from build123d import *

# Parameters (mm, degrees)
SKETCH1_W           = 165
SKETCH1_H           = 50
BOSS_EXTRUDE1_DEPTH = 2.5
FILLET1_R           = 25
SKETCH2_R           = 2.5
CUT_EXTRUDE1_DEPTH  = 2.5
SKETCH3_R           = 2.5
CUT_EXTRUDE2_DEPTH  = 2.5
SKETCH4_R           = 2.25
BOSS_EXTRUDE2_DEPTH = 8
SKETCH6_R           = 1.5
CUT_EXTRUDE4_DEPTH  = 87.841810207


with BuildPart() as part:
    # Sketch1 → Boss-Extrude1 (new body)
    with BuildSketch(Plane.XY):
        Rectangle(SKETCH1_W, SKETCH1_H)
    extrude(amount=BOSS_EXTRUDE1_DEPTH)

    # Fillet1
    fillet1_edges = [part.edges().sort_by_distance(p)[0] for p in [
        (-82.5, -25, 1.25),
        (-82.5, 25, 1.25),
        (82.5, -25, 1.25),
        (82.5, 25, 1.25),
    ]]
    fillet(fillet1_edges, radius=FILLET1_R - 0.0001)  # a hair under: the kernel refuses the full size

    # Sketch2 → Cut-Extrude1 (cut)
    with BuildSketch(Plane.XY.offset(2.5)):
        with Locations((-5, 16)):
            Circle(SKETCH2_R)
        with Locations((5, 16)):
            Circle(SKETCH2_R)
    cut_extrude1 = extrude(amount=-CUT_EXTRUDE1_DEPTH, mode=Mode.SUBTRACT)

    # Mirror1: Cut-Extrude1 across plane
    add(cut_extrude1.mirror(Plane.ZX), mode=Mode.SUBTRACT)

    # Sketch3 → Cut-Extrude2 (cut)
    with BuildSketch(Plane(origin=(0, 0, 0), x_dir=(-1, 0, 0), z_dir=(0, 0, -1))):
        with Locations((-57.5, 0)):
            Circle(SKETCH3_R)
    extrude(amount=-CUT_EXTRUDE2_DEPTH, mode=Mode.SUBTRACT)

    # Sketch4 → Boss-Extrude2 (add)
    with BuildSketch(Plane.XY.offset(2.5)):
        with Locations(Location((-57.5, 0, 0), (0, 0, 180))):
            Circle(SKETCH4_R)
    extrude(amount=BOSS_EXTRUDE2_DEPTH)

    # Sketch6 → Cut-Extrude4 (cut, through all)
    with BuildSketch(Plane(origin=(0, 0, 0), x_dir=(-1, 0, 0), z_dir=(0, 0, -1))):
        with Locations((-25, 18.5)):
            Circle(SKETCH6_R)
        with Locations((25, 18.5)):
            Circle(SKETCH6_R)
    extrude(amount=-CUT_EXTRUDE4_DEPTH, mode=Mode.SUBTRACT)


solid = part.part
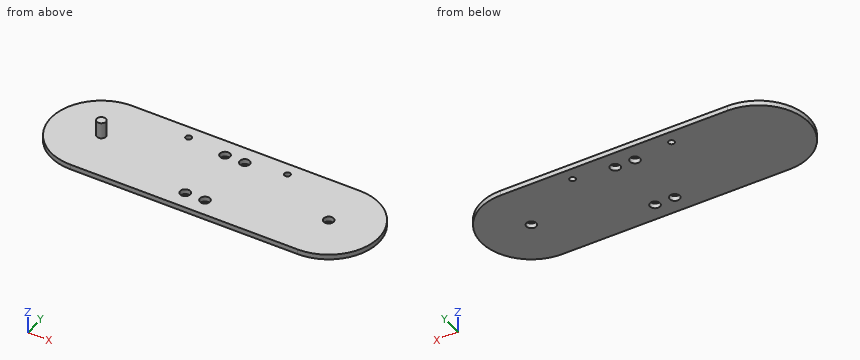
Could you check a few things on this model? Use its own coordinates, in mm. Round coordinates to 2 decimals unless told otherwise and drop trailing zeros. Write each loop counter-clockwise with the first axis right and the second up, starting at its lowest first coordinate (ties: lowest second). Pieces come first, ordered by that corner, then holes. Notation, with made-up numbers: (87, -6) - (128, -6) arc R23 cw to (128, 24) - close; hole circle Ø4 at (78, 34.5). An arc over 180 degrees is marked (long way). Use a Markdown table: item, result.
Q1. I want a section at D-D (x = 39). List the corners of the cut face in (y, z) for me.
Output values:
| item | result |
|---|---|
| outline | (-25, 0) - (25, 0) - (25, 2.5) - (-25, 2.5) - close |
Q2. For pin 1 (3 mm diameter, centred on x = 52, y = -17.5, fed in from +Z); pin 2 (3 mm diameter, centred on x = 5, y = -16, fed in from -Z); pin 3 (5 mm diameter, centred on x = -63.5, z = 1, fed in from -Y), each with a flat end and sliding along its axis, tell me the tip position at first contact or that it passes through.
Output values:
| item | result |
|---|---|
| pin 1 | z = 2.5 |
| pin 2 | through |
| pin 3 | y = -24.75 |
Q3. I want a section at B-B (x = -25). List the corners of the cut face in (y, z) for me.
Output values:
| item | result |
|---|---|
| outline | (-25, 0) - (17, 0) - (17, 2.5) - (-25, 2.5) - close; (20, 0) - (25, 0) - (25, 2.5) - (20, 2.5) - close |
Q4. Please list where these lines run through material, in increasing order: L1, parallel to Y at x = 5, z = 1.15; L2, parallel to Y at x = -25, z = 1.1; L3, parallel to X at y = -14, z = 1.75.
Output values:
| item | result |
|---|---|
| L1 | -25 to -18.5, -13.5 to 13.5, 18.5 to 25 |
| L2 | -25 to 17, 20 to 25 |
| L3 | -78.21 to -6.5, -3.5 to 3.5, 6.5 to 78.21 |
Q5. I want a section at C-C (z = 4). List the corners of the cut face in (x, y) for me.
Output values:
| item | result |
|---|---|
| outline | circle Ø4.5 at (-57.5, 0) |
Q6. I want a section at A-A (x = -5). List the corners of the cut face in (y, z) for me.
Output values:
| item | result |
|---|---|
| outline | (-25, 0) - (-18.5, 0) - (-18.5, 2.5) - (-25, 2.5) - close; (-13.5, 0) - (13.5, 0) - (13.5, 2.5) - (-13.5, 2.5) - close; (18.5, 0) - (25, 0) - (25, 2.5) - (18.5, 2.5) - close |
